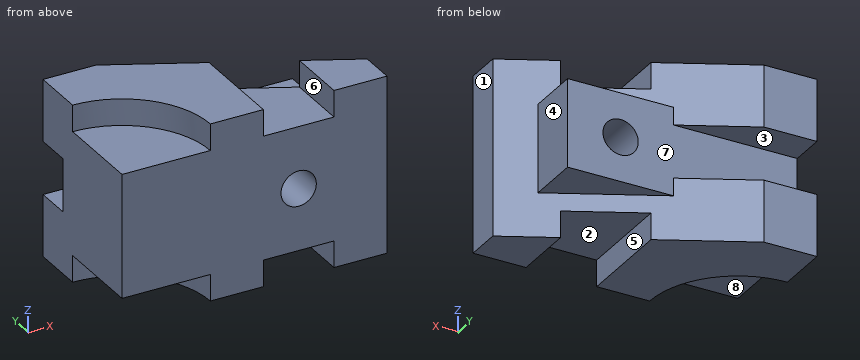
```python
from build123d import *

# Parameters (mm, degrees)
BOSS_EXTRUDE1_DEPTH = 100
SKETCH2_R           = 50
CUT_EXTRUDE1_DEPTH  = 15
SKETCH3_R           = 50
CUT_EXTRUDE2_DEPTH  = 15
SKETCH4_W           = 40
SKETCH4_H           = 15
CUT_EXTRUDE3_DEPTH  = 75
SKETCH5_W           = 60
SKETCH5_H           = 50
BOSS_EXTRUDE2_DEPTH = 60
SKETCH7_W           = 30
SKETCH7_H           = 20
CUT_EXTRUDE4_DEPTH  = 100
SKETCH8_R           = 10
CUT_EXTRUDE5_DEPTH  = 100


with BuildPart() as part:
    # Sketch1 → Boss-Extrude1 (new body)
    with BuildSketch(Plane.XY):
        Polygon((-52.06185567, 38.608247423), (-52.06185567, -41.391752577), (97.93814433, -41.391752577), (97.93814433, -21.391752577), (-22.06185567, 38.608247423), align=None)
    extrude(amount=-BOSS_EXTRUDE1_DEPTH)

    # Sketch2 → Cut-Extrude1 (cut)
    with BuildSketch(Plane.XY):
        with Locations((-52.06185567, -41.391752577)):
            Circle(SKETCH2_R)
    extrude(amount=-CUT_EXTRUDE1_DEPTH, mode=Mode.SUBTRACT)

    # Sketch3 → Cut-Extrude2 (cut)
    with BuildSketch(Plane(origin=(0, 0, -100), x_dir=(-1, 0, 0), z_dir=(0, 0, -1))):
        with Locations((52.06185567, -41.391752577)):
            Circle(SKETCH3_R)
    extrude(amount=-CUT_EXTRUDE2_DEPTH, mode=Mode.SUBTRACT)

    # Sketch4 → Cut-Extrude3 (cut)
    with BuildSketch(Plane.XZ.offset(41.391752577)):
        with Locations((47.93814433, -7.5)):
            Rectangle(SKETCH4_W, SKETCH4_H)
        with Locations((47.93814433, -92.5)):
            Rectangle(SKETCH4_W, SKETCH4_H)
    extrude(amount=-CUT_EXTRUDE3_DEPTH, mode=Mode.SUBTRACT)

    # Sketch5 → Boss-Extrude2 (add)
    with BuildSketch(Plane.XZ.offset(41.391752577)):
        with Locations((47.93814433, -50)):
            Rectangle(SKETCH5_W, SKETCH5_H)
    extrude(amount=-BOSS_EXTRUDE2_DEPTH)

    # Sketch7 → Cut-Extrude4 (cut)
    with BuildSketch(Plane.ZY.offset(52.06185567)):
        with Locations((-50, 28.608247423)):
            Rectangle(SKETCH7_W, SKETCH7_H)
    extrude(amount=-CUT_EXTRUDE4_DEPTH, mode=Mode.SUBTRACT)

    # Sketch8 → Cut-Extrude5 (cut)
    with BuildSketch(Plane(origin=(0, 18.608247423, 0), x_dir=(1, 0, 0), z_dir=(0, 1, 0))):
        with Locations((47.93814433, 50)):
            Circle(SKETCH8_R)
    extrude(amount=-CUT_EXTRUDE5_DEPTH, mode=Mode.SUBTRACT)


solid = part.part
```
Model file for the job. Use its own axes, mm. Face numbers are marked on the shaded views. A direction names the side the tool comes from. Coordinates: 2 decimals unless noted, no trailing zeros. Loops run counter-clockwise (first coordinate to the right, second up) from the corner with the lowest first, then second, coordinate; pieces in that order, holes last. Notation, with made-up numbers: (-2.75, 68) -> (2.25, 68) arc R22 ccw to (2.25, 84) -> close; hole circle Ø7 at (58, 78.5). An arc over 180 degrees is marked (long way). Answer as a JSON object with one key per item and string values.
Q1. Cut at A-A (z = -50). List the corners of the cut face in (x, y), and give its area (3 significant figures).
Report:
{"outline": "(-52.06, -41.39) -> (37.94, -41.39) -> (37.94, 18.61) -> (-52.06, 18.61) -> close; (57.94, -41.39) -> (97.94, -41.39) -> (97.94, -21.39) -> (77.94, -11.39) -> (77.94, 18.61) -> (57.94, 18.61) -> close", "area": "7,100 mm2"}
Q2. Pull direction Z, two halves, no side cores. Call the marked faces 1, 2 and 3: released by +Z, released by -Z, zero draft, split by the parting line, or undercut.
Report:
{"face 1": "zero draft", "face 2": "released by -Z", "face 3": "undercut"}
Q3. Probe probe 1 along X at (y, z) = (-26, -50); probe 2 along Z at (x, y) = (-28, 31); probe 3 along X at (y, z) = (4.5, -50). List the from-to ranges inside material, lowest first.
Report:
{"probe 1": "x = -52.06 to 37.94, 57.94 to 97.94", "probe 2": "z = -100 to -65, -35 to 0", "probe 3": "x = -52.06 to 37.94, 57.94 to 77.94"}
Q4. Cut at D-D (x = 24). List the corners of the cut face in (y, z), and give its area (3 significant figures).
Report:
{"outline": "(-41.39, -100) -> (15.58, -100) -> (15.58, -75) -> (18.61, -75) -> (18.61, -25) -> (15.58, -25) -> (15.58, 0) -> (-41.39, 0) -> close", "area": "5,850 mm2"}
Q5. Cut at C-C (z = -37.5). List the corners of the cut face in (x, y).
Report:
{"outline": "(-52.06, -41.39) -> (97.94, -41.39) -> (97.94, -21.39) -> (77.94, -11.39) -> (77.94, 18.61) -> (-52.06, 18.61) -> close"}
Q6. Cut at B-B (y = 21). List the corners of the cut face in (x, z).
Report:
{"outline": "(-52.06, -100) -> (13.15, -100) -> (13.15, -65) -> (-52.06, -65) -> close; (-52.06, -35) -> (13.15, -35) -> (13.15, 0) -> (-52.06, 0) -> close"}
Q7. Flat gauge pins, fed straight in: P1, Ø16.5, axis at y = -5, z = -7.5, coming from the +X side; P2, Ø2, axis at x = -18.5, y = -16, coming from the -Z side; P3, Ø9, axis at y = 5.5, z = -51.5, coming from the +X side; P4, Ø16, axis at x = -32.5, y = 23.5, coming from the +Z side. Where does each tip first touch, or does it go through?
Report:
{"P1": "stops at x = 81.65", "P2": "stops at z = -85", "P3": "stops at x = 77.94", "P4": "stops at z = 0"}
Q8. 3-axis set-ups, long thin cutter, end or side, ignore diameter. For the marked faces 4, 5, 6, 7 and 8: which of +Z, -Z, +X, -X, +Y, -Y reach the whole face in a straight line?
Report:
{"face 4": "+Z, -Z, +X, +Y", "face 5": "-Z, +Y, -Y", "face 6": "+Z, +Y, -Y", "face 7": "+X, +Y", "face 8": "-Z, -X, -Y"}
